Verification items for the finished model (mm, model axes). Face numbers are marked on the shaded views. A direction names the side the tool comes from. Coordinates: 2 decimals unless noted, no trailing zeros. Write each loop counter-clockwise with the first axis right and the second up, starting at its lowest first coordinate (ties: lowest second). Pieces come first, ordered by that corner, then holes. Notation, with made-up numbers: (64.5, 65) -> (94.5, 65) arc R25 cw to (94.5, 83) -> close; hole circle Ø4 at (35.5, -13). An arc over 180 degrees is marked (long way). Write each question's results on one line, items separated by ' | '. Start each with the question number.
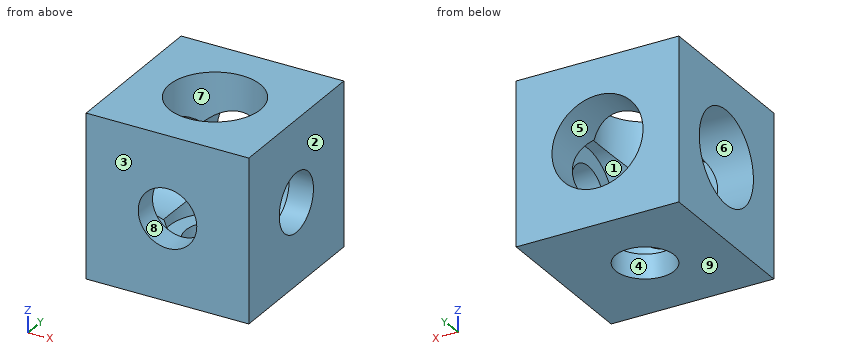
Autodesk Inventor part; units mm, degrees
ref_plane "YZ Plane" through (0, 0, 0) normal (1, 0, 0) x (0, 1, 0)
ref_plane "XZ Plane" through (0, 0, 0) normal (0, 1, 0) x (-1, 0, 0)
ref_plane "XY Plane" through (0, 0, 0) normal (0, 0, 1) x (1, 0, 0)
sketch "Sketch1" plane through (0, 0, 0) normal (1, 0, 0) x (0, 1, 0)
  line L0 (0, 0) -> (20, 0)
  line L1 (20, 0) -> (20, -20)
  line L2 (20, -20) -> (0, -20)
  line L3 (0, -20) -> (0, 0)
  dimension "d0" = 20
  dimension "d1" = 20
extrude "Extrusion1" add sketch "Sketch1" along normal blind 20
sketch "Sketch2" plane through (0, 0, 0) normal (0, 0, 1) x (1, 0, 0)
  circle A0 centre (10, 10) radius 3.6
  line L0 (0, 20) -> (0, 0)
  line L1 (0, 20) -> (20, 20)
  dimension "d4" = 10
  dimension "d5" = 10
  dimension "d6" = 7.2
extrude "Extrusion2" cut sketch "Sketch2" against normal blind 20
sketch "Sketch3" plane through (20, 0, 0) normal (1, 0, 0) x (0, 0, -1)
  circle A0 centre (10, 10) radius 3.6
  line L0 (20, 20) -> (0, 20)
  line L1 (0, 20) -> (0, 0)
  dimension "d9" = 10
  dimension "d10" = 10
  dimension "d11" = 7.2
extrude "Extrusion3" cut sketch "Sketch3" against normal blind 20
sketch "Sketch4" plane through (0, 20, 0) normal (0, 1, 0) x (1, 0, 0)
  line L0 (13.6, 6.4) -> (10, 10)
  circle A0 centre (10, 10) radius 3.6
  line L1 (20, 20) -> (20, 0)
  line L2 (0, 0) -> (20, 0)
  dimension "d14" = 7.2
  dimension "d15" = 10
  dimension "d16" = 10
extrude "Extrusion4" cut sketch "Sketch4" against normal blind 20
sketch "Sketch5" plane through (0, 0, 0) normal (-1, 0, 0) x (0, 0, 1)
  circle A0 centre (-10, 10) radius 3.6
  circle A1 centre (-10, 10) radius 5.7
  point P0 (0, 0)
  dimension "d19" = 11.4
extrude "Extrusion5" cut sketch "Sketch5" against normal blind 17 contours A0 | A1
sketch "Sketch6" plane through (0, 0, 0) normal (0, 0, 1) x (1, 0, 0)
  circle A0 centre (10, 10) radius 3.6
  circle A1 centre (10, 10) radius 5.6
  point P0 (0, 0)
  dimension "d22" = 11.2
extrude "Extrusion6" cut sketch "Sketch6" against normal blind 17 contours A0 | A1
sketch "Sketch7" plane through (0, 20, 0) normal (0, 1, 0) x (1, 0, 0)
  circle A0 centre (10, 10) radius 3.6
  circle A1 centre (10, 10) radius 5.6
  point P0 (0, 0)
  dimension "d25" = 11.2
extrude "Extrusion7" cut sketch "Sketch7" against normal blind 17 contours A0 | A1
properties part number "2020CubeConnector" material "Aluminum 6061-AHC"
1. Sectioned sample at D-D on z = -14.75. Record the cut outline in (x, y).
2. Depth check by flat-ended pin: pin 1 Ø5.5 at (x, y) = (11, 12.5) entering from +Z; pin 2 Ø9 at (x, z) = (10.5, -10) entering from +Y; pin 3 Ø5.5 at (y, z) = (10.5, -8.5) entering from -X. Enter the tip coordinate at first touch or a pass-through.
3. Sectioned sample at B-B on x = 10. Record the cut outline in (y, z).
4. Sectioned sample at A-A on z = -10. Record the cut outline in (x, y).
5. Sectioned sample at C-C on x = 14.5. Record the cut outline in (y, z).
6. Tool access check on the marked faces 5, 6, 7, 8 and 9. Record the directions out of +Z, -Z, +X, -X, +Y, -Y that give a thin tool (end or side, any length) a straight path to the whole face; none if there is none.
7. Material ranges on probe 1 along Y at (x, z) = (3.5, -10); probe 2 along X at (y, z) = (10, -2.3); probe 3 along Z at (x, y) = (10, 17), recorded low to high. Write a range as from..to.
8. Mould release check, pull along Y, two halves, no side actions. Record for the marked faces 1, 2, 3 and 4: +Y half, -Y half, draft (parallel to the pull), parting line (faces both ways), or undercut.
Computed values:
1) outline: (0, 0) -> (20, 0) -> (20, 20) -> (12.97, 20) -> (12.97, 14.75) arc R5.6 cw to (14.63, 13.15) -> (17, 13.15) -> (17, 6.85) -> (14.63, 6.85) arc R5.6 cw to (12.97, 5.25) -> (12.97, 3) -> (7.03, 3) -> (7.03, 5.25) arc R5.6 cw to (5.37, 6.85) -> (0, 6.85) -> close; (0, 13.15) -> (5.37, 13.15) arc R5.6 cw to (7.03, 14.75) -> (7.03, 20) -> (0, 20) -> close
2) pin 1: stops at z = -17 | pin 2: stops at y = 3 | pin 3: stops at x = 17
3) outline: (0, -20) -> (6.4, -20) -> (6.4, -17) -> (4.4, -17) -> (4.4, -15.6) -> (3, -15.6) -> (3, -13.6) -> (0, -13.6) -> close; (0, -6.4) -> (3, -6.4) -> (3, -4.4) -> (4.4, -4.4) -> (4.4, 0) -> (0, 0) -> close; (13.6, -20) -> (20, -20) -> (20, -15.6) -> (15.6, -15.6) -> (15.6, -17) -> (13.6, -17) -> close; (15.6, -4.4) -> (20, -4.4) -> (20, 0) -> (15.6, 0) -> close
4) outline: (0, 0) -> (6.4, 0) -> (6.4, 3) -> (4.4, 3) -> (4.4, 4.3) -> (0, 4.3) -> close; (0, 15.7) -> (4.4, 15.7) -> (4.4, 20) -> (0, 20) -> close; (13.6, 0) -> (20, 0) -> (20, 6.4) -> (17, 6.4) -> (17, 4.3) -> (15.6, 4.3) -> (15.6, 3) -> (13.6, 3) -> close; (15.6, 15.7) -> (17, 15.7) -> (17, 13.6) -> (20, 13.6) -> (20, 20) -> (15.6, 20) -> close
5) outline: (0, -20) -> (20, -20) -> (20, -13.33) -> (14.62, -13.33) arc R5.7 cw to (13.33, -14.62) -> (13.33, -17) -> (6.67, -17) -> (6.67, -14.62) arc R5.7 cw to (5.38, -13.33) -> (3, -13.33) -> (3, -6.67) -> (5.38, -6.67) arc R5.7 cw to (6.67, -5.38) -> (6.67, 0) -> (0, 0) -> close; (13.33, -5.38) arc R5.7 cw to (14.62, -6.67) -> (20, -6.67) -> (20, 0) -> (13.33, 0) -> close
6) face 5: +Y | face 6: -X | face 7: +Z | face 8: +Y, -Y | face 9: -Z, +X, -X, +Y, -Y
7) probe 1: y = 0..4.3, 15.7..20 | probe 2: x = 0..4.4, 15.6..20 | probe 3: z = -20..-15.6, -4.4..0
8) face 1: undercut | face 2: draft | face 3: -Y half | face 4: undercut
